Source: three-view drawing plus pictorial views. Frame: mm from the lowest corner of the part. Coordinates: 2 decimals unless noted, no trailing zeros. Write each loop counter-clockwise with the first axis right and the second up, starting at its lowest first coordinate (ties: lowest second). Pieces come first, ordered by that corner, then holes. Notation, with made-up numbers: M 32,-26 L 76,-26 A15 cw 76,-10 Z; hole C -13,57 d8. An arc over 180 degrees is marked long. Use CSV: the item, a comma, the result in double quotes.
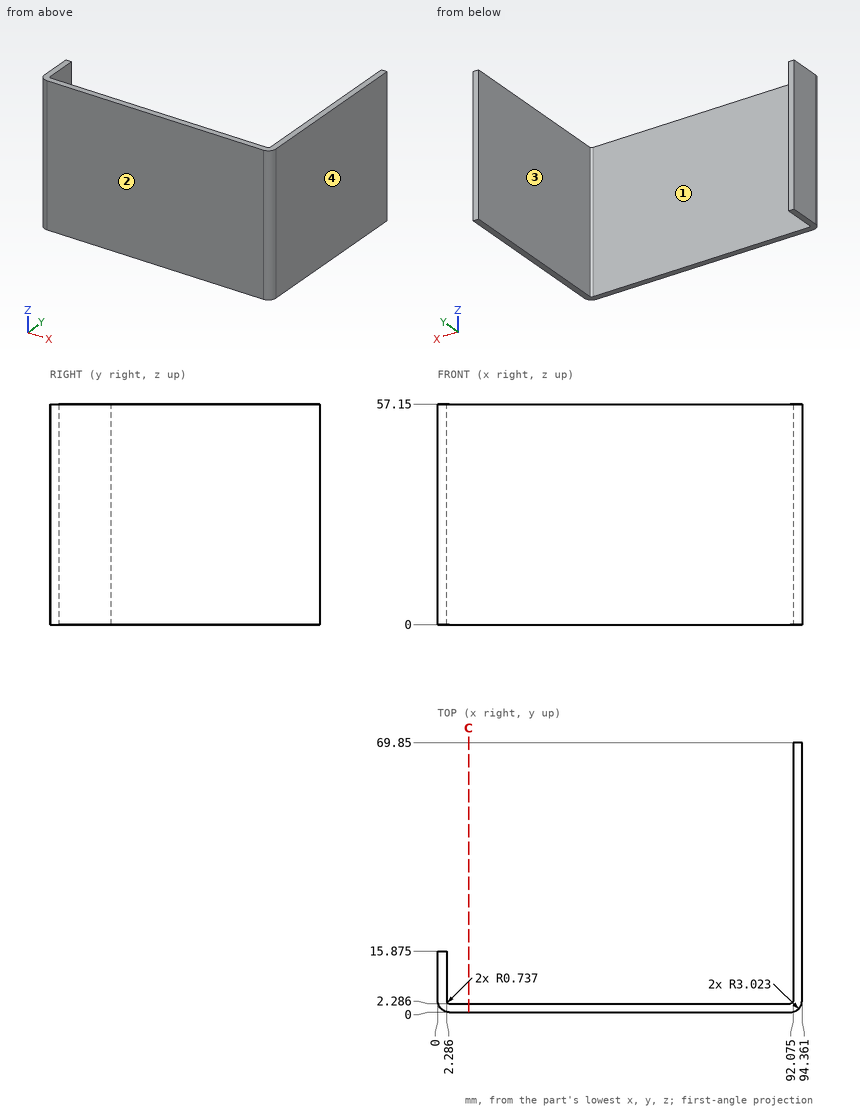
1. Contact query for flat-ended pins moving along their axis: pin 1 Ø0.7 at (x, z) = (0.5, 27) entering from +Y (3 decimals); pin 2 Ø1 at (x, z) = (30.5, 49.5) entering from +Y. Output: stop coordinate, or through.
Resolved:
pin 1,"stops at y = 15.875"
pin 2,"stops at y = 2.29"
2. Material intervals for line 1 (Y direction, x = 56, z = 4); line 2 (X direction, y = 20.5, z = 50) (1 decimal); line 3 (X direction, y = 5.5, z = 11.5) (1 decimal), sorted ascending. Write a range as [from, to].
Resolved:
line 1,"y = [0, 2.29]"
line 2,"x = [92.1, 94.4]"
line 3,"x = [0, 2.3], [92.1, 94.4]"
3. Section C-C (x = 8). Return loops of the section in (y, z), then the cut area to 3 significant figures.
Resolved:
outline,"M 0,0 L 2.29,0 L 2.29,57.15 L 0,57.15 Z"
area,"131 mm^2"
4. Mould query, pull axis X, two halves, no side actions, for the marked faces 1, 2, 3 and 4. Classes: pulls with the +X half, pulls with the -X half, needs draft (parallel to the pull), parting line crosses it, or undercut.
Resolved:
face 1,"undercut"
face 2,"needs draft"
face 3,"undercut"
face 4,"pulls with the +X half"
